```python
from build123d import *

# Parameters (mm, degrees)
BOSS_EXTRUDE1_DEPTH = 30
SKETCH2_R           = 125
CUT_EXTRUDE1_DEPTH  = 5.35
SKETCH3_W           = 10
SKETCH3_H           = 5
CUT_EXTRUDE2_DEPTH  = 5
CHAMFER2_SIZE       = 8
FILLET1_R           = 20


with BuildPart() as part:
    # Sketch1 → Boss-Extrude1 (new body)
    with BuildSketch(Plane(origin=(0, 0, 0), x_dir=(1, 0, 0), z_dir=(0, 1, 0))):
        with BuildLine():
            Line((-114.748366001, 66.25), (-106.088111964, 61.25))
            ThreePointArc((-106.088111964, 61.25), (-106.088111964, -61.25), (0, -122.5))
            Line((0, -122.5), (0, -132.5))
            ThreePointArc((0, -132.5), (-114.748366001, -66.25), (-114.748366001, 66.25))
        make_face()
    extrude(amount=BOSS_EXTRUDE1_DEPTH)

    # Sketch2 → Cut-Extrude1 (cut)
    with BuildSketch(Plane(origin=(0, 0, 0), x_dir=(1, 0, 0), z_dir=(0, 1, 0))):
        Circle(SKETCH2_R)
    extrude(amount=CUT_EXTRUDE1_DEPTH, mode=Mode.SUBTRACT)

    # Sketch3 → Cut-Extrude2 (cut)
    with BuildSketch(Plane.XY.offset(132.5)):
        with Locations((-5, 15)):
            Rectangle(SKETCH3_W, SKETCH3_H)
        Polygon((-15, 22.5), (-15, 7.5), (-10, 12.5), (-10, 17.5), align=None)
    cut_extrude2 = extrude(amount=-CUT_EXTRUDE2_DEPTH, mode=Mode.SUBTRACT)

    # Mirror1: Cut-Extrude2 across plane
    add(cut_extrude2.mirror(Plane(origin=(0, 0, 0), x_dir=(-0.8660254037844389, 0, 0.4999999999999995), z_dir=(0.4999999999999996, 0, 0.8660254037844389))), mode=Mode.SUBTRACT)

    # Chamfer2
    # the kernel refuses this chamfer: 8 mm, written as the material it takes off along each edge
    with BuildSketch(Plane(origin=(0, 30, 0), x_dir=(0.1547578410621492, 0, 0.9879524333842102), z_dir=(0.9879524333842102, 0, -0.1547578410621492))) as chamfer2_piece_1:
        Polygon((132.5 - CHAMFER2_SIZE, 0), (132.5, CHAMFER2_SIZE), (132.5, 0), align=None)
    revolve(axis=Axis((0, 30, 0), (0, -1, 0)), revolution_arc=137.805504207, mode=Mode.SUBTRACT)

    # Fillet1
    # the kernel refuses this fillet: 20 mm, written as the material it takes off along each edge
    with BuildSketch(Plane(origin=(0, 22, 0), x_dir=(0.04293180283805991, 0, 0.9990780051152532), z_dir=(0.9990780051152532, 0, -0.04293180283805991))) as fillet1_piece_1:
        with BuildLine():
            CenterArc((132.5 - FILLET1_R, FILLET1_R * 0.414213562373), FILLET1_R, 315, 45)
            Line((132.5, FILLET1_R * 0.414213562373), (132.5, 0))
            Line((132.5, 0), (132.5 - FILLET1_R * 0.292893218813, -FILLET1_R * 0.292893218813))
        make_face()
    revolve(axis=Axis((0, 22, 0), (0, -1, 0)), revolution_arc=124.921134732, mode=Mode.SUBTRACT)


solid = part.part
```
For this review, take the finished solid that the model builds, in its own axes (mm). A direction names the side the tool comes from. Give positions to 0.01 mm unless a question says otherwise; leave off trailing zeros. Write each loop counter-clockwise with the first axis right and the second up, starting at its lowest first coordinate (ties: lowest second). Pieces come first, ordered by that corner, then holes. Notation, with made-up numbers: M 8,66.25 L 48,66.25 A23 ccw 48,86.25 Z; hole C -4,69 d7. An arc over 180 degrees is marked long. Answer as a JSON object with one key per item and string values. Group by question number.
Item 1: Consider section B-B on y = 20.5. Write out the cut boundary in (x, z).
Item 2: For probe 1 along X at (y, z) = (12, 2); probe 2 along Z at (x, y) = (-54, 26); probe 3 along X at (y, z) = (5.5, -52), list the stretches that pass through material, from the lowest coordinate up. Write a range as [from, to].
Item 3: For pin 1 Ø6 at (x, y) = (-72.5, 21.5) entering from -Z; pin 2 Ø12 at (y, z) = (22, -22.5) entering from -X; pin 3 Ø1 at (x, y) = (-85, 20) entering from +Z; pin 4 Ø4.5 at (x, z) = (-116.5, -61.5) entering from -Y, all flat-tipped, find the tip position at first contact; note any pin that passes through.
Item 4: Tool access review of faces 5 (the flat face through (-118.7, 10, -54.1)), 6 (the flat face through (-5, 17.5, 130)), 7 (the flat face through (-9, 15, 127.5)), 8 (the flat face through (-115, 12.5, -61)), 9 (the cylindrical face through (-109.158, 2.638, 60.906)): name each direction out of +Z, -Z, +X, -X, +Y, -Y from which nothing blocks a thin tool from reaching the whole face with its end or side.
Item 5: Consider section C-C on y = 2. Write out the cut boundary in (x, z).
Item 6: Consider section A-A on y = 10.5. Write out the cut boundary in (x, z).
Item 7: Draft analysis for pull direction Y (two halves, no side actions). For faces 1 (the flat face through (-110, 0, 62)), 2 (the flat face through (-12.5, 10, 129.8)), 3 (the flat face through (-5, 12.5, 130)), 4 (the flat face through (0, 15, 127)), state which applies: +Y half, -Y half, draft (parallel to the pull), parting line (faces both ways), or undercut.
Check result:
{
 "1": {"outline": "M -120.48,-52.24 L -117.92,-50.76 L -116.92,-52.49 L -119.66,-54.08 A131.31 ccw -113.72,-65.66 L -106.09,-61.25 A122.5 cw 0,122.5 L 0,131.31 A131.31 ccw -13,130.67 L -13,127.5 L -15,127.5 L -15,130.45 A131.31 ccw Z"},
 "2": {"probe 1": "x = [-132.48, -122.48]", "probe 2": "z = [109.96, 116.36]", "probe 3": "x = [-121.87, -110.92]"},
 "3": {"pin 1": "stops at z = 96.47", "pin 2": "stops at x = -130.84", "pin 3": "stops at z = 100.79", "pin 4": "stops at y = 0"},
 "4": {"face 5": "none", "face 6": "+Z, +X", "face 7": "+Z", "face 8": "-Z, -X", "face 9": "+X, -Y"},
 "5": {"outline": "M -114.75,-66.25 L -108.25,-62.5 A125 cw 0,125 L 0,132.5 A132.5 ccw Z"},
 "6": {"outline": "M -121.51,-52.83 L -117.92,-50.76 L -116.42,-53.36 L -120.28,-55.59 A132.5 ccw -114.75,-66.25 L -106.09,-61.25 A122.5 cw 0,122.5 L 0,132.5 A132.5 ccw -12,131.96 L -12,127.5 L -15,127.5 L -15,131.65 A132.5 ccw Z"},
 "7": {"face 1": "-Y half", "face 2": "undercut", "face 3": "undercut", "face 4": "draft"}
}
